Source: CAD feature listing. Evaluate the final solid. Frame: model axes, mm. Face numbers are marked on the shaded views. A direction names the side the tool comes from. Give positions to 0.01 mm unless a question says otherwise; leave off trailing zeros. Loops run counter-clockwise (first coordinate to the right, second up) from the corner with the lowest first, then second, coordinate; pieces in that order, holes last.
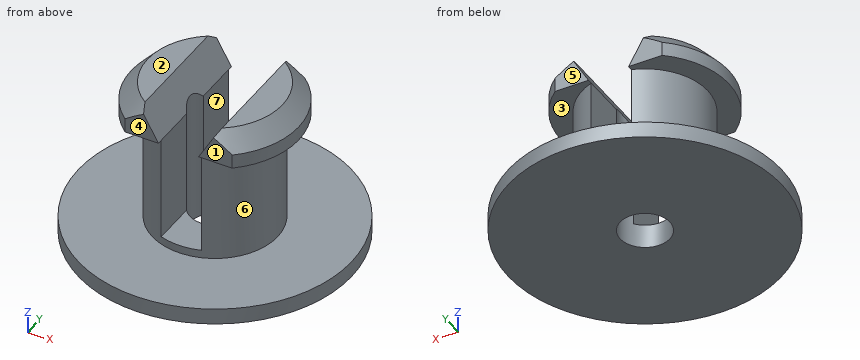
```python
from build123d import *

# Parameters (mm, degrees)
SKETCH1_R                = 8.5
BOSS_EXTRUDE1_DEPTH      = 6
BOSS_EXTRUDE1_DEPTH_BACK = 4.5
SKETCH2_R                = 8.5
SKETCH2_R_2              = 3.9
CUT_EXTRUDE1_DEPTH       = 3.5
CUT_EXTRUDE1_DEPTH_BACK  = 3.5
SKETCH3_R                = 8.5
SKETCH3_R_2              = 6
CUT_EXTRUDE2_DEPTH       = 3.5
CUT_EXTRUDE4_DEPTH       = 3.5
CUT_EXTRUDE5_DEPTH       = 8.5
SKETCH10_R               = 1.55
CUT_EXTRUDE6_DEPTH       = 10
CUT_EXTRUDE7_DEPTH       = 8


with BuildPart() as part:
    # Sketch1 → Boss-Extrude1 (new body, two sides)
    with BuildSketch(Plane.XY) as boss_extrude1_sk:
        Circle(SKETCH1_R)
    extrude(amount=BOSS_EXTRUDE1_DEPTH)
    extrude(boss_extrude1_sk.sketch, amount=-BOSS_EXTRUDE1_DEPTH_BACK)

    # Sketch2 → Cut-Extrude1 (cut, two sides)
    with BuildSketch(Plane.XY) as cut_extrude1_sk:
        Circle(SKETCH2_R)
        Circle(SKETCH2_R_2, mode=Mode.SUBTRACT)
    extrude(amount=CUT_EXTRUDE1_DEPTH, mode=Mode.SUBTRACT)
    extrude(cut_extrude1_sk.sketch, amount=-CUT_EXTRUDE1_DEPTH_BACK, mode=Mode.SUBTRACT)

    # Sketch3 → Cut-Extrude2 (cut)
    with BuildSketch(Plane(origin=(0, 0, 3.5), x_dir=(-1, 0, 0), z_dir=(0, 0, -1))):
        Circle(SKETCH3_R)
        Circle(SKETCH3_R_2, mode=Mode.SUBTRACT)
    extrude(amount=-CUT_EXTRUDE2_DEPTH, mode=Mode.SUBTRACT)

    # Sketch6 → Cut-Revolve1 (revolve, cut)
    with BuildSketch(Plane(origin=(0, 0, 0), x_dir=(0, 0, -1), z_dir=(1, 0, 0))):
        Polygon((-5.5, 0), (-5.5, 4.2), (-4.379199334, 5.208720599), (-3.5, 5.208720599), (-3.5, 6), (-6, 6), (-6, 0), align=None)
    revolve(axis=Axis((0, 0, -5.814918194), (0, 0, 1)), mode=Mode.SUBTRACT)

    # Sketch8 → Cut-Extrude4 (cut)
    with BuildSketch(Plane(origin=(0, 0, 3.5), x_dir=(-1, 0, 0), z_dir=(0, 0, -1))):
        Polygon((-10, 4), (0, 4), (10, 4), (10, 8.647445608), (-10, 8.647445608), align=None)
        Polygon((10, -4), (0, -4), (-10, -4), (-10, -8.418803799), (10, -8.418803799), align=None)
    extrude(amount=-CUT_EXTRUDE4_DEPTH, mode=Mode.SUBTRACT)

    # Sketch9 → Cut-Extrude5 (cut)
    with BuildSketch(Plane.XY.offset(5.5)):
        Polygon((0, 4), (-1.25, 4), (-1.25, -4), (1.25, -4), (1.25, 4), align=None)
    extrude(amount=-CUT_EXTRUDE5_DEPTH, mode=Mode.SUBTRACT)

    # Sketch10 → Cut-Extrude6 (cut)
    with BuildSketch(Plane(origin=(0, 0, -4.5), x_dir=(-1, 0, 0), z_dir=(0, 0, -1))):
        Circle(SKETCH10_R)
    extrude(amount=-CUT_EXTRUDE6_DEPTH, mode=Mode.SUBTRACT)

    # Sketch12 → Cut-Extrude7 (cut)
    with BuildSketch(Plane(origin=(0, 4, 0), x_dir=(1, 0, 0), z_dir=(0, 1, 0))):
        Polygon((-1.25, -3.5), (-1.25, -5.5), (-2.4, -5.5), align=None)
        Polygon((1.25, -5.5), (2.4, -5.5), (1.25, -3.5), align=None)
    extrude(amount=-CUT_EXTRUDE7_DEPTH, mode=Mode.SUBTRACT)


solid = part.part
```
(1) Section B-B, the plane x = 0. Return the cut outline in (y, z).
A:
outline: (-8.5, -4.5) - (-1.55, -4.5) - (-1.55, -3) - (-3.9, -3) - (-3.9, -3.5) - (-8.5, -3.5) - close; (1.55, -4.5) - (8.5, -4.5) - (8.5, -3.5) - (3.9, -3.5) - (3.9, -3) - (1.55, -3) - close
(2) Section D-D, the plane y = 5.5. Return the cut outline in (x, z).
A:
outline: (-6.48, -4.5) - (6.48, -4.5) - (6.48, -3.5) - (-6.48, -3.5) - close
(3) Reachability of the marked faces 4, 5, 6 and 7 from +Z, -Z, +X, -X, +Y, -Y: full face, straight path, thin tool, end or side. Return the list, or none.
A:
face 4: +Z, +X, -X, -Y
face 5: +Z, +X, -X, +Y
face 6: none
face 7: +Z, +Y, -Y
(4) Section A-A, the plane y = 0. Return the cut outline in (x, z).
A:
outline: (-8.5, -4.5) - (-1.55, -4.5) - (-1.55, 4.02) - (-2.4, 5.5) - (-4.2, 5.5) - (-5.21, 4.38) - (-5.21, 3.5) - (-3.9, 3.5) - (-3.9, -3.5) - (-8.5, -3.5) - close; (1.55, -4.5) - (8.5, -4.5) - (8.5, -3.5) - (3.9, -3.5) - (3.9, 3.5) - (5.21, 3.5) - (5.21, 4.38) - (4.2, 5.5) - (2.4, 5.5) - (1.55, 4.02) - close
(5) First-contact query: pin 1 (2 mm diameter, centred on x = 1, z = 0, fed in from -Y); pin 2 (4 mm diameter, centred on y = -2.5, z = -3.5, fed in from +X); pin 3 (5 mm diameter, centred on y = -4.5, z = 0.5, fed in from +X). Flat tips, straight axial feed; report the tip coordinate or a pass-through.
A:
pin 1: stops at y = -3.69
pin 2: stops at x = 8.49
pin 3: stops at x = 3.35
(6) Ray query, line 1 along X through (y, z) = (0, 0); line 2 along Z through (x, y) = (5.5, 3); line 3 along X through (y, z) = (1, -1). Return the intervals inside material, ascending.
A:
line 1: x = -3.9 to -1.55, 1.55 to 3.9
line 2: z = -4.5 to -3.5
line 3: x = -3.77 to -1.25, 1.25 to 3.77
(7) Mould query, pull axis Z, two halves, no side actions, for the marked faces 1, 2 and 3. Classes: pulls with the +Z half, pulls with the -Z half, needs draft (parallel to the pull), parting line crosses it, or undercut.
A:
face 1: needs draft
face 2: pulls with the +Z half
face 3: undercut
(8) Section C-C, the plane z = 3. Return the cut outline in (x, y), then the cut area to 3 significant figures.
A:
outline: (-1.25, -3.69) - (-1.25, -0.92) arc R1.55 cw to (-1.25, 0.92) - (-1.25, 3.69) arc R3.9 ccw to start; (1.25, -3.69) arc R3.9 ccw to (1.25, 3.69) - (1.25, 0.92) arc R1.55 cw to (1.25, -0.92) - close
area: 27.9 mm2
